Geometry check sheet. Reference: the model listing, model coordinates, mm. Give positions to 0.01 mm unless a question says otherwise; leave off trailing zeros. Order: outer loops, then holes, each group sorted by start corner. A loop starts at its lowest first (then second) coordinate and runs counter-clockwise, first axis right, second up.
from build123d import *

# Parameters (mm, degrees)
F0_R     = 1.651
F1_DEPTH = 1.7
F1_TAPER = -41
F3_DEPTH = 17.35
F4_SIZE2 = 1.5877132403
F4_SIZE  = 2.75
F6_DEPTH = 0.5


with BuildPart() as f1:
    # F0 (on Top) → F1 (new body)
    with BuildSketch(Plane.XY):
        Circle(F0_R)
    extrude(amount=F1_DEPTH, taper=F1_TAPER)

    # F3 (add, through all): a face of the model
    f3_faces = [f1.faces().sort_by_distance(p)[0] for p in [
        (0, 0, 0),
    ]]
    extrude(f3_faces, amount=F3_DEPTH)

    # F4
    f4_edges = [f1.edges().sort_by_distance(p)[0] for p in [
        (-1.651, 0, -17.35),
    ]]
    f4_side = f1.faces().sort_by_distance((-1.651, 0, -8.675))[0]
    chamfer(f4_edges, length=F4_SIZE, length2=F4_SIZE2, reference=f4_side)

    # F5 (on face) → F6 (cut)
    with BuildSketch(Plane.XY.offset(1.7)):
        Polygon((-0.3023856843, -2.3319076281), (0, -2.3434136529), (0.2844197443, -2.3434136529), (0.2844197443, -0.4104074033), (1.9527882105, -0.4104074033), (1.9527882105, 0.40651788), (0.2729137486, 0.2569399949), (0.2729137486, 1.7987425672), (-0.3023856843, 1.7987425672), (-0.3023856843, 0.3950118844), (-1.8441881984, 0.3950118844), (-1.8441881984, -0.3298654919), (-0.3023856843, -0.3298654919), align=None)
    extrude(amount=-F6_DEPTH, mode=Mode.SUBTRACT)


solid = f1.part
Item 1: Gauge pin test, flat ends, axial feed: pin 1 (0.6 mm diameter, centred on y = 1, z = 1.5, fed in from -X); pin 2 (3 mm diameter, centred on y = -2, z = -6.5, fed in from -X); pin 3 (3 mm diameter, centred on x = -1, z = -14, fed in from -Y). Record the tip position at first contact, or that the pin passes through.
Reported:
pin 1: stops at x = -3.03
pin 2: stops at x = -1.57
pin 3: stops at y = -1.65
Item 2: Scan lines: L1, parallel to Z at x = -1, y = -2.5; L2, parallel to Y at x = -0.25, z = -7.5; L3, parallel to X at y = 0.5, z = -3.5. Record each from-to range of solid material in increasing order.
Reported:
L1: z = 1.2 to 1.7
L2: y = -1.63 to 1.63
L3: x = -1.57 to 1.57
Item 3: Sectioned sample at A-A (z = -13). Enter the section's corners in (x, y), and give its area (3 significant figures).
Reported:
outline: circle Ø3.3 at (0, 0)
area: 8.56 mm2
Item 4: Sectioned sample at B-B (z = -15.75). Enter the section's corners in (x, y).
Reported:
outline: circle Ø1.97 at (0, 0)
Item 5: Draft check along Y on faces 1 (the flat face through (0, 0, 1.2)), 2 (the cylindrical face through (1.525, -0.632, -7.198)), 3 (the flat face through (1, -1, 1.7)). Enter one of: released by +Y, released by -Y, zero draft, split by the parting line, or undercut.
Reported:
face 1: undercut
face 2: split by the parting line
face 3: zero draft
